from build123d import *

# Parameters (mm, degrees)
SKETCH1_W           = 3.5
SKETCH1_H           = 14.5
BOSS_EXTRUDE1_DEPTH = 0.37
SKETCH2_W           = 2.48
SKETCH2_H           = 8.81
BOSS_EXTRUDE2_DEPTH = 0.56
SKETCH3_W           = 0.07
SKETCH3_H           = 10
BOSS_EXTRUDE3_DEPTH = 0.03
SKETCH5_W           = 1.8
SKETCH5_H           = 7.79
BOSS_EXTRUDE4_DEPTH = 0.45
BOSS_EXTRUDE5_DEPTH = 7.79


with BuildPart() as part:
    # Sketch1 → Boss-Extrude1 (new body)
    with BuildSketch(Plane.XY):
        Rectangle(SKETCH1_W, SKETCH1_H)
    extrude(amount=BOSS_EXTRUDE1_DEPTH)

    # Sketch2 → Boss-Extrude2 (add)
    with BuildSketch(Plane.XY.offset(0.37)):
        with Locations((0, -2.285)):
            Rectangle(SKETCH2_W, SKETCH2_H)
        Polygon((0.59, -6.69), (-0.59, -6.69), (-0.59, -7.22), (-0.47, -7.22), (0.47, -7.22), (0.59, -7.22), align=None)
        Polygon((0.463655834, -7.25), (-0.463655834, -7.25), (-0.41, -7.503725219), (0.41, -7.503725219), align=None)
        Polygon((0.47, -7.22), (-0.47, -7.22), (-0.463655834, -7.25), (0.463655834, -7.25), align=None)
    extrude(amount=BOSS_EXTRUDE2_DEPTH)

    # Sketch3 → Boss-Extrude3 (add)
    with BuildSketch(Plane.XY.offset(0.93)):
        with Locations((-0.375, -12.503725219)):
            Rectangle(SKETCH3_W, SKETCH3_H)
        with Locations((-0.125, -12.503725219)):
            Rectangle(SKETCH3_W, SKETCH3_H)
        with Locations((0.125, -12.503725219)):
            Rectangle(SKETCH3_W, SKETCH3_H)
        with Locations((0.375, -12.503725219)):
            Rectangle(SKETCH3_W, SKETCH3_H)
    extrude(amount=-BOSS_EXTRUDE3_DEPTH)

    # Sketch5 → Boss-Extrude4 (add)
    with BuildSketch(Plane.XY.offset(0.93)):
        with Locations((0, -2.795)):
            Rectangle(SKETCH5_W, SKETCH5_H)
    extrude(amount=BOSS_EXTRUDE4_DEPTH)

    # Sketch6 → Boss-Extrude5 (add)
    with BuildSketch(Plane.XZ.offset(6.69)):
        Polygon((-0.52, 1.38), (-0.9, 1.76), (0.9, 1.76), (0.52, 1.38), align=None)
    extrude(amount=-BOSS_EXTRUDE5_DEPTH)


solid = part.part
Design review of the part built by this model. Coordinates are the model's own, in mm. A direction names the side the tool comes from. Coordinates: 2 decimals unless noted, no trailing zeros. Write each loop counter-clockwise with the first axis right and the second up, starting at its lowest first coordinate (ties: lowest second). Pieces come first, ordered by that corner, then holes. Notation, with made-up numbers: (88, 24) - (121, 24) arc R13 ccw to (121, 30) - close; hole circle Ø5 at (-1.5, 35). An arc over 180 degrees is marked (long way). Use one line per item in the form item = value.
Q1. Consider section C-C (y = 3.5). Write out the cut boundary in (x, z), plus the area to 4 significant figures.
Taken from the geometry:
outline = (-1.75, 0) - (1.75, 0) - (1.75, 0.37) - (-1.75, 0.37) - close
area = 1.295 mm^2
Q2. Machinability: for faces 1 (the flat face through (0, 1.1, 1.3)), 2 (the flat face through (0, 0, 0)), which of the approach directions +Z, -Z, +X, -X, +Y, -Y give a long, thin tool a straight path to every point of the face, cutting with its end or side? Answer none if there is none.
Taken from the geometry:
face_1 = +Z, +X, -X, +Y
face_2 = -Z, +X, -X, +Y, -Y
Q3. For probe 1 along Z at (x, y) = (1.6, 1); probe 2 along Y at (x, z) = (1.55, 0.25); probe 3 along X at (y, z) = (1, 0.75), list the stretches that pass through material, from the lowest coordinate up.
Taken from the geometry:
probe_1 = 0 to 0.37
probe_2 = -7.25 to 7.25
probe_3 = -1.24 to 1.24
Q4. Consider section B-B (y = -2.25). Write out the cut boundary in (x, z), plus the area to 3 significant figures.
Taken from the geometry:
outline = (-1.75, 0) - (1.75, 0) - (1.75, 0.37) - (1.24, 0.37) - (1.24, 0.93) - (0.9, 0.93) - (0.9, 1.38) - (0.52, 1.38) - (0.9, 1.76) - (-0.9, 1.76) - (-0.52, 1.38) - (-0.9, 1.38) - (-0.9, 0.93) - (-1.24, 0.93) - (-1.24, 0.37) - (-1.75, 0.37) - close
area = 4.03 mm^2
Q5. Consider section A-A (y = -15). Count the separate pieces of the cut face and the enclosed holes in it, plus the area to 3 significant figures.
Taken from the geometry:
separate_pieces = 4
enclosed_holes = 0
area = 0.00840 mm^2
Q6. Insertion check: pin 1 Ø2 at (x, y) = (1.5, -10) entering from -Z; pin 2 Ø1 at (x, y) = (1.5, 5) entering from -Z; pin 3 Ø0.9 at (x, y) = (0, -11.5) entering from +Z; pin 4 Ø2 at (x, y) = (0, -10) entering from -Z. Each pin has a flat end and moves straight along its axis. Give the tip position at first contact, or say it passes through.
Taken from the geometry:
pin_1 = through
pin_2 = 0
pin_3 = 0.93
pin_4 = 0.9
